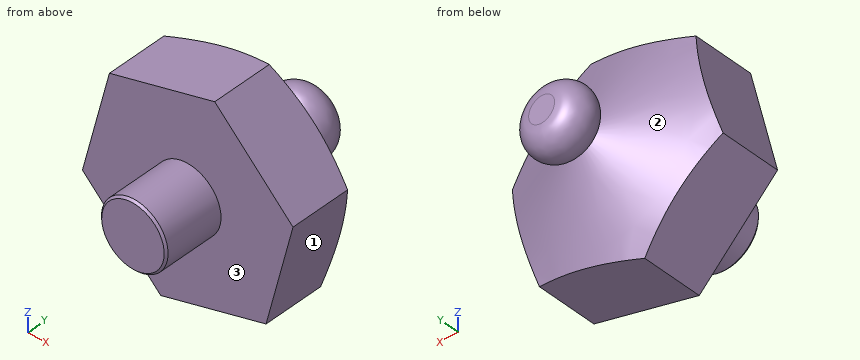
```python
from build123d import *

# Parameters (mm, degrees)
SKETCH2_OUTSIDE_W  = 146.052
SKETCH2_OUTSIDE_H  = 146.052
CUT_EXTRUDE1_DEPTH = 126.665925527
CHAMFER1_SIZE      = 1


with BuildPart() as part:
    # Sketch1 → Revolve1 (revolve)
    with BuildSketch(Plane.XY, mode=Mode.PRIVATE) as revolve1_sk:
        with BuildLine():
            Line((0, 100), (-6.380027739, 100))
            ThreePointArc((-6.380027739, 100), (-16.380027739, 90), (-6.380027739, 80))
            Line((-6.380027739, 80), (-53.814147018, 58.94590846))
            Line((-53.814147018, 58.94590846), (-53.814147018, 29.542302358))
            Line((-53.814147018, 29.542302358), (-16.380027739, 29.542302358))
            Line((-16.380027739, 29.542302358), (-16.380027739, 0))
            Line((-16.380027739, 0), (0, 0))
            Line((0, 0), (0, 100))
        make_face()
    revolve(revolve1_sk.sketch.rotate(Axis((0, 0, 0), (0, 1, 0)), 270), axis=Axis((0, 0, 0), (0, 1, 0)))

    # Sketch2 outside → Cut-Extrude1 (cut, through all)
    with BuildSketch(Plane(origin=(0, 100, 0), x_dir=(1, 0, 0), z_dir=(0, 1, 0))):
        Rectangle(SKETCH2_OUTSIDE_W, SKETCH2_OUTSIDE_H)
        Polygon((-38.527261507, -37.5714325), (13.274184248, -52.151303453), (51.801445755, -14.579870953), (38.527261507, 37.5714325), (-13.274184248, 52.151303453), (-51.801445755, 14.579870953), align=None, mode=Mode.SUBTRACT)
    extrude(amount=-CUT_EXTRUDE1_DEPTH, mode=Mode.SUBTRACT)

    # Chamfer1
    chamfer1_edges = [part.edges().sort_by_distance(p)[0] for p in [
        (0, 0, 16.380027739),
    ]]
    chamfer(chamfer1_edges, length=CHAMFER1_SIZE)


solid = part.part
```
Check sheet for the modelled part. Datum: model origin and axes. Units: mm. Face numbers are marked on the shaded views. A direction names the side the tool comes from. Round coordinates to 2 decimals unless told otherwise and drop trailing zeros. Order: outer loops, then holes, each group sorted by start corner. A loop starts at its lowest first (then second) coordinate and runs counter-clockwise, first axis right, second up. Notation, with made-up numbers: M 23.25,59.25 L 54.25,59.25 A18 cw 54.25,94.25 Z; hole C 88.25,83.25 d9. An arc over 180 degrees is marked long. Answer in a Markdown table with one row per item.
(1) Gauge pin test, flat ends, axial feed: pin 1 (10 mm diameter, centred on y = 74, z = -10.5, fed in from -X); pin 2 (5 mm diameter, centred on x = -28, z = -2, fed in from +Y); pin 3 (1.5 mm diameter, centred on y = 73.5, z = -6.5, fed in from -X). Record the tip position at first contact, or that the pin passes through.
Findings:
| item | result |
|---|---|
| pin 1 | stops at x = -29.46 |
| pin 2 | stops at y = 71.48 |
| pin 3 | stops at x = -21.78 |
(2) Section check B-B on y = 17.5. Record the boundary of the cut face in (x, z).
Findings:
| item | result |
|---|---|
| outline | C 0,0 d32.76 |
(3) Section check A-A on y = 32. Record the boundary of the cut face in (x, z), plus the area to 3 significant figures.
Findings:
| item | result |
|---|---|
| outline | M -51.8,-14.58 L -13.27,-52.15 L 38.53,-37.57 L 51.8,14.58 L 13.27,52.15 L -38.53,37.57 Z |
| area | 7,520 mm^2 |
(4) Material ranges on line 1 along Y through (x, z) = (-18, -39); line 2 along X through (y, z) = (6, -7); line 3 along Z through (x, y) = (6, 73.5), recorded low to high. Write a range as from..to.
Findings:
| item | result |
|---|---|
| line 1 | y = 29.54..63.77 |
| line 2 | x = -14.81..14.81 |
| line 3 | z = -20.15..20.15 |
(5) Set-up check for the marked faces 1, 2 and 3: record each of +Z, -Z, +X, -X, +Y, -Y from which the full face is reachable in a straight line by a thin tool's end or side.
Findings:
| item | result |
|---|---|
| face 1 | -Z, +X, +Y, -Y |
| face 2 | none |
| face 3 | -Y |
